```python
from build123d import *

# Parameters (mm, degrees)
F0_W     = 13.97
F0_H     = 12.7
F0_W_2   = 10.16
F0_H_2   = 8.255
F1_DEPTH = 5.08
F2_R     = 8.89
F3_DEPTH = 3.175
F4_SIZE  = 0.762
F6_DEPTH = 10.16


with BuildPart() as f1:
    # F0 (on Front) → F1 (new body)
    with BuildSketch(Plane.XZ):
        with Locations((0, -3.175)):
            Rectangle(F0_W, F0_H)
        with Locations((0, -3.4925)):
            Rectangle(F0_W_2, F0_H_2, mode=Mode.SUBTRACT)
    extrude(amount=F1_DEPTH)

    # F2 (on face) → F3 (join)
    with BuildSketch(Plane.XY.offset(3.175)):
        with Locations((0, -2.292242)):
            Circle(F2_R)
    extrude(amount=F3_DEPTH)

    # F4
    f4_edges = [f1.edges().sort_by_distance(p)[0] for p in [
        (-8.89, -2.292242, 6.35),
    ]]
    chamfer(f4_edges, length=F4_SIZE)

    # F5 (on face) → F6 (join)
    with BuildSketch(Plane(origin=(5.08, 0, 0), x_dir=(0, -1, 0), z_dir=(-1, 0, 0))):
        Polygon((0, -7.62), (5.08, -7.62), (4.064, -6.35), (3.302, -7.3025), (2.54, -6.35), (1.778, -7.3025), (1.016, -6.35), align=None)
    extrude(amount=F6_DEPTH)


solid = f1.part
```
Can you work these out from the model? Positions are in its coordinate system, mm. A direction names the side the tool comes from. Coordinates: 2 decimals unless noted, no trailing zeros. Loops run counter-clockwise (first coordinate to the right, second up) from the corner with the lowest first, then second, coordinate; pieces in that order, holes last. Notation, with made-up numbers: M -38,-36 L 4,-36 A8 ccw 4,-27 Z; hole C -21.75,81 d11. An arc over 180 degrees is marked long. Put each result on its own line as item: value. Start each with the question number.
(1) I need wall thicknesses on probe 1 along X at (y, z) = (-2.25, -2.75) (3 decimals); probe 2 along Y at (x, z) = (5.5, 0.25); probe 3 along Z at (x, y) = (-4, -8) (3 decimals). Which ranges of each line are inside material? Lowest first, please.
(2) Imagine slicing it at A-A on z = -4. List the corners of the cut face in (x, y) for me (3 decimals), and give its area (3 significant figures).
(3) We'd pull the mould along Z, two halves only. Please class faces 1 (the face through (-1.93, -10.97, 4.36)), 2 (the face through (0, -3, -9.525)), 3 (the face through (0, -2, 6.35)), 4 (the face through (5.08, -3, -4)): +Z half, -Z half, draft (parallel to the pull), parting line (faces both ways), or undercut.
(4) Will these pins go through, and if not, where does the flat tip stop? pin 1 Ø6 at (x, z) = (1, 4.5) entering from -Y; pin 2 Ø5.5 at (y, z) = (-1.5, -2.5) entering from -X (3 decimals); pin 3 Ø4 at (y, z) = (-3, -4.5) entering from +X (3 decimals); pin 4 Ø3 at (y, z) = (-4.5, 2) entering from +X.
(5) Which directions (+Z, -Z, +X, -X, +Y, -Y) give clear straight access to the entire face, cutting with the end or side of a thin tool? Please do faces 5 (the face through (0.071, -0.515, -6.976)), 6 (the face through (0.07, -1.4, -6.83)), 7 (the face through (0, 0, 1)).
Worked answers:
1. probe 1: x = -6.985 to -5.08, 5.08 to 6.985
1. probe 2: y = -5.08 to 0
1. probe 3: z = 3.175 to 6.35
2. outline: M -6.985,-5.08 L -5.08,-5.08 L -5.08,0 L -6.985,0 Z; M 5.08,-5.08 L 6.985,-5.08 L 6.985,0 L 5.08,0 Z
2. area: 19.4 mm2
3. face 1: draft
3. face 2: -Z half
3. face 3: +Z half
3. face 4: undercut
4. pin 1: stops at y = -11.18
4. pin 2: stops at x = -6.985
4. pin 3: stops at x = 6.985
4. pin 4: stops at x = 8.8
5. face 5: +Y
5. face 6: none
5. face 7: -Z, +X, -X, +Y
